Geometry: final body of the model. Coordinates: model frame, mm. A direction names the side the tool comes from. Coordinates: 2 decimals unless noted, no trailing zeros. Order: outer loops, then holes, each group sorted by start corner. A loop starts at its lowest first (then second) coordinate and runs counter-clockwise, first axis right, second up. Notation, with made-up numbers: (77.5, 50.5) -> (131.5, 50.5) arc R29 ccw to (131.5, 78.5) -> close; hole circle Ø11 at (82, -10). An arc over 180 degrees is marked (long way). Answer in a Markdown table with one row per item. Add a question column.
1) Section query A-A on z = 0. Return the cut outline in (x, y), then the cut area to 3 significant figures.
2) Section query C-C on y = 0. Return the cut outline in (x, z).
3) Set-up query: faces 1 (the face through (3.68, 0.53, 11.99)), 2 (the face through (1, 0, 13)), 3 (the face through (-18, -14, 0)), 4 (the face through (-18, 0, 4)), 5 (the face through (-18, 0, -4)). Return all of +Z, -Z, +X, -X, +Y, -Y with unobstructed straight access to the full face (end or side cutting, diameter ignored); none if empty.
4) Section query D-D on x = -11.5. Return the cut outline in (y, z).
5) Ray query, line 1 (Y direction, x = 1.55, z = 9.5); line 2 (Y direction, x = 1.7, z = -9.5); line 3 (Y direction, x = -11, z = -3.75). Return the intervals inside material, ascending. Write a range as from..to.
6) Contact query for flat-ended pins moving along their axis: P1, Ø12, axis at x = -2.5, z = -5.5, coming from the -Y side; P2, Ø1.5, axis at x = -29.5, y = 11.5, coming from the +Z side; P3, Ø9, axis at x = -23.5, z = 1, coming from the -Y side; P4, Ø3, axis at y = -12, z = 9.5, coming from the -X side. Output: stop coordinate, or through.
7) Section query B-B on z = -8.75. Return the cut outline in (x, y), then the cut area to 3 significant figures.
8) Pull-direction query (Y, two-part tool) for faces 6 (the face through (5.1, 0, 0)), 7 (the face through (1.1, -10.5, 8.6)), 8 (the face through (-18, 14, 0)), 9 (the face through (1, -15.5, 0)); classes: +Y half, -Y half, draft (parallel to the pull), parting line (faces both ways), or undercut.
```python
from build123d import *

# Parameters (mm, degrees)
SKETCH2_W           = 26
SKETCH2_H           = 31
SKETCH2_R           = 1.75
BOSS_EXTRUDE1_DEPTH = 2.3
SKETCH3_R           = 12
BOSS_EXTRUDE2_DEPTH = 2.8
SKETCH4_W           = 8
SKETCH4_H           = 28
BOSS_EXTRUDE3_DEPTH = 37


with BuildPart() as part:
    # Sketch2 → Boss-Extrude1 (new body)
    with BuildSketch(Plane(origin=(0, 0, 0), x_dir=(0, 0, -1), z_dir=(1, 0, 0))):
        Rectangle(SKETCH2_W, SKETCH2_H)
        with Locations((-9.5, -12)):
            Circle(SKETCH2_R, mode=Mode.SUBTRACT)
        with Locations((9.5, 12)):
            Circle(SKETCH2_R, mode=Mode.SUBTRACT)
    extrude(amount=BOSS_EXTRUDE1_DEPTH)

    # Sketch3 → Boss-Extrude2 (add)
    with BuildSketch(Plane(origin=(2.3, 0, 0), x_dir=(0, 0, -1), z_dir=(1, 0, 0))):
        Circle(SKETCH3_R)
    extrude(amount=BOSS_EXTRUDE2_DEPTH)

    # Sketch4 → Boss-Extrude3 (add)
    with BuildSketch(Plane.ZY):
        Rectangle(SKETCH4_W, SKETCH4_H)
    extrude(amount=BOSS_EXTRUDE3_DEPTH)


solid = part.part
```
Result:
| question | item | result |
|---|---|---|
| 1 | outline | (-37, -14) -> (0, -14) -> (0, -15.5) -> (2.3, -15.5) -> (2.3, -12) -> (5.1, -12) -> (5.1, 12) -> (2.3, 12) -> (2.3, 15.5) -> (0, 15.5) -> (0, 14) -> (-37, 14) -> close |
| 1 | area | 1,170 mm2 |
| 2 | outline | (-37, -4) -> (0, -4) -> (0, -13) -> (2.3, -13) -> (2.3, -12) -> (5.1, -12) -> (5.1, 12) -> (2.3, 12) -> (2.3, 13) -> (0, 13) -> (0, 4) -> (-37, 4) -> close |
| 3 | face 1 | +X |
| 3 | face 2 | +Z, +X, -X, +Y, -Y |
| 3 | face 3 | +Z, -Z, -X, -Y |
| 3 | face 4 | +Z, -X, +Y, -Y |
| 3 | face 5 | -Z, -X, +Y, -Y |
| 4 | outline | (-14, -4) -> (14, -4) -> (14, 4) -> (-14, 4) -> close |
| 5 | line 1 | -15.5..-13.75, -10.25..15.5 |
| 5 | line 2 | -15.5..10.25, 13.75..15.5 |
| 5 | line 3 | -14..14 |
| 6 | P1 | y = -15.5 |
| 6 | P2 | z = 4 |
| 6 | P3 | y = -14 |
| 6 | P4 | through |
| 7 | outline | (0, -15.5) -> (2.3, -15.5) -> (2.3, -8.21) -> (5.1, -8.21) -> (5.1, 8.21) -> (2.3, 8.21) -> (2.3, 10.42) -> (0, 10.42) -> close; (0, 13.58) -> (2.3, 13.58) -> (2.3, 15.5) -> (0, 15.5) -> close |
| 7 | area | 110 mm2 |
| 8 | face 6 | draft |
| 8 | face 7 | undercut |
| 8 | face 8 | +Y half |
| 8 | face 9 | -Y half |
